Input: dimensioned drawing with shaded views. Units: mm. Origin: part minimum x, y, z. A direction names the side the tool comes from. Round coordinates to 2 decimals unless told otherwise and drop trailing zeros. Loops run counter-clockwise (first coordinate to the right, second up) from the corner with the lowest first, then second, coordinate; pieces in that order, holes last. Notation, with made-up numbers: M 83.25,-37.5 L 104.25,-37.5 A27 cw 104.25,-12.5 Z; hole C 25,-19 d4. An arc over 180 degrees is marked long. Write each question's results on one line, items separated by ' | '. Start each with the question number.
1. Contact query for flat-ended pins moving along their axis: pin 1 Ø1 at (y, z) = (10, 17.5) entering from +X; pin 2 Ø2.5 at (x, z) = (11, 19) entering from -Y; pin 3 Ø1 at (y, z) = (7, 15) entering from +X; pin 4 Ø6 at (y, z) = (6.5, 13.5) entering from -X. Output: stop coordinate, or through.
2. Ray query, line 1 (Z direction, x = 11, y = 11); line 2 (Y direction, x = 6.5, z = 16); line 3 (Z direction, x = 13.5, y = 12.5). Return the intervals inside material, ascending.
3. Set-up query: the marked faces 5 and 6. Return all of +Z, -Z, +X, -X, +Y, -Y with unobstructed straight access to the full face (end or side cutting, diameter ignored); none if empty.
4. Section C-C on x = 3. Output: boundary loops of the cut face in (y, z).
5. Section D-D on y = 9. Output: boundary loops of the cut face in (x, z), and give its area (3 significant figures).
6. Section B-B on z = 19. Output: boundary loops of the cut face in (x, y).
7. Section A-A on x = 10.5. Output: boundary loops of the cut face in (y, z).
8. Draft query along X for the marked faces 1, 2, 3 and 4. Return one class per face: released by +X, released by -X, zero draft, split by the parting line, or undercut.
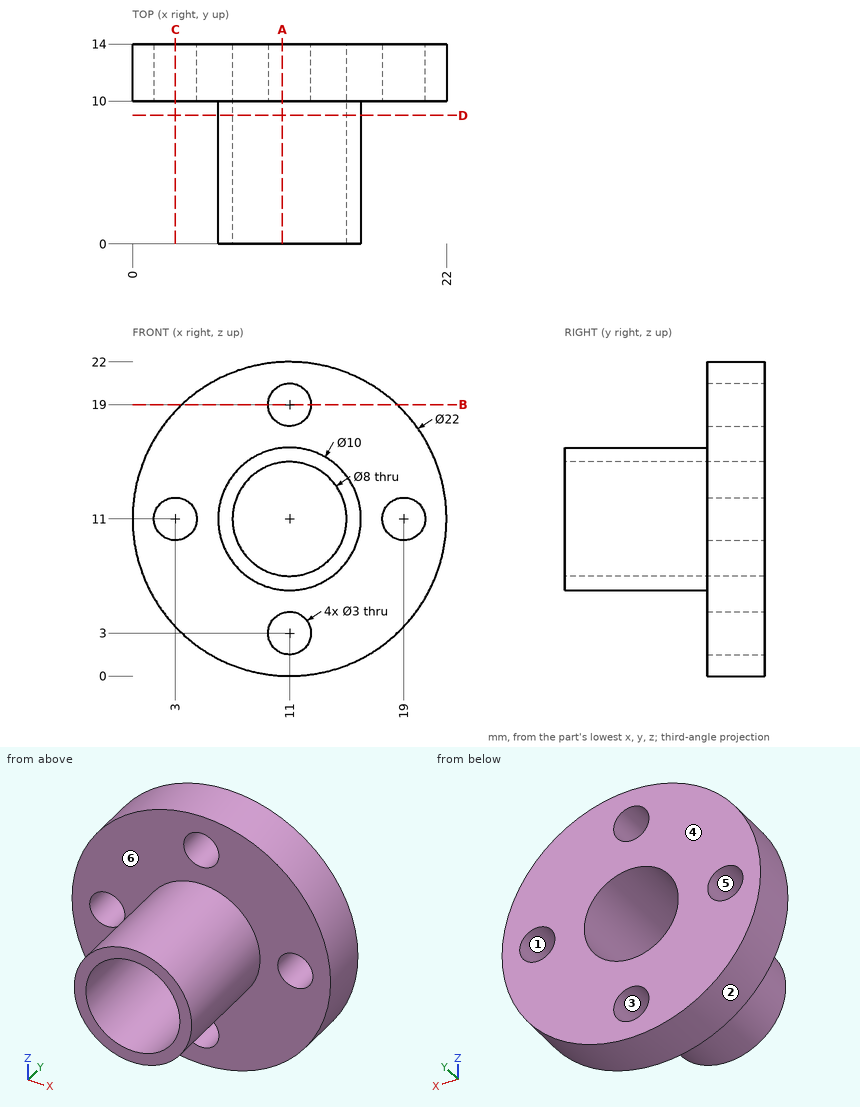
Taken from the geometry:
1) pin 1: x = 20.22 | pin 2: through | pin 3: x = 14.57 | pin 4: x = 6
2) line 1: 0 to 1.5, 4.5 to 7, 15 to 17.5, 20.5 to 22 | line 2: 10 to 14 | line 3: 0.29 to 7.88, 14.12 to 21.71
3) face 5: +Y, -Y | face 6: -Y
4) outline: M 10,3.45 L 14,3.45 L 14,9.5 L 10,9.5 Z; M 10,12.5 L 14,12.5 L 14,18.55 L 10,18.55 Z
5) outline: C 11,11 d10; hole C 11,11 d8 | area: 28.3 mm^2
6) outline: M 3.45,10 L 9.5,10 L 9.5,14 L 3.45,14 Z; M 12.5,10 L 18.55,10 L 18.55,14 L 12.5,14 Z
7) outline: M 0,6.03 L 10,6.03 L 10,4.41 L 14,4.41 L 14,7.03 L 0,7.03 Z; M 0,14.97 L 14,14.97 L 14,17.59 L 10,17.59 L 10,15.97 L 0,15.97 Z; M 10,0.01 L 14,0.01 L 14,1.59 L 10,1.59 Z; M 10,20.41 L 14,20.41 L 14,21.99 L 10,21.99 Z
8) face 1: undercut | face 2: split by the parting line | face 3: undercut | face 4: zero draft
